Input: dimensioned drawing with shaded views. Units: mm. Origin: part minimum x, y, z. Coordinates: 2 decimals unless noted, no trailing zeros. Loops run counter-clockwise (first coordinate to the right, second up) from the corner with the lowest first, then second, coordinate; pieces in that order, holes last.
(1) Section A-A, the plane z = 21. Return loops of the section in (x, y) (1 decimal), then the cut area to 3 significant figures.
(2) Section C-C, the plane y = 2.65. Return loops of the section in (x, z) (1 decimal), then the cut area to 3 significant figures.
(3) Line query: L1, parallel to X at y = 2.6, z = 26; L2, parallel to X at y = 0.7, z = 24.5 (1 decimal); L3, parallel to Y at x = 32, z = 2. Output: solid intervals per line, ascending.
(4) Contact query for flat-ended pins moving along their axis: P1, Ø1.5, axis at y = 1.5, z = 5.5, coming from the +X side; P2, Ø1.1, axis at y = 2.5, z = 50, coming from the -X side. Output: stop coordinate, or through.
(5) Section B-B, the plane x = 47. Return loops of the section in (y, z) (1 decimal).
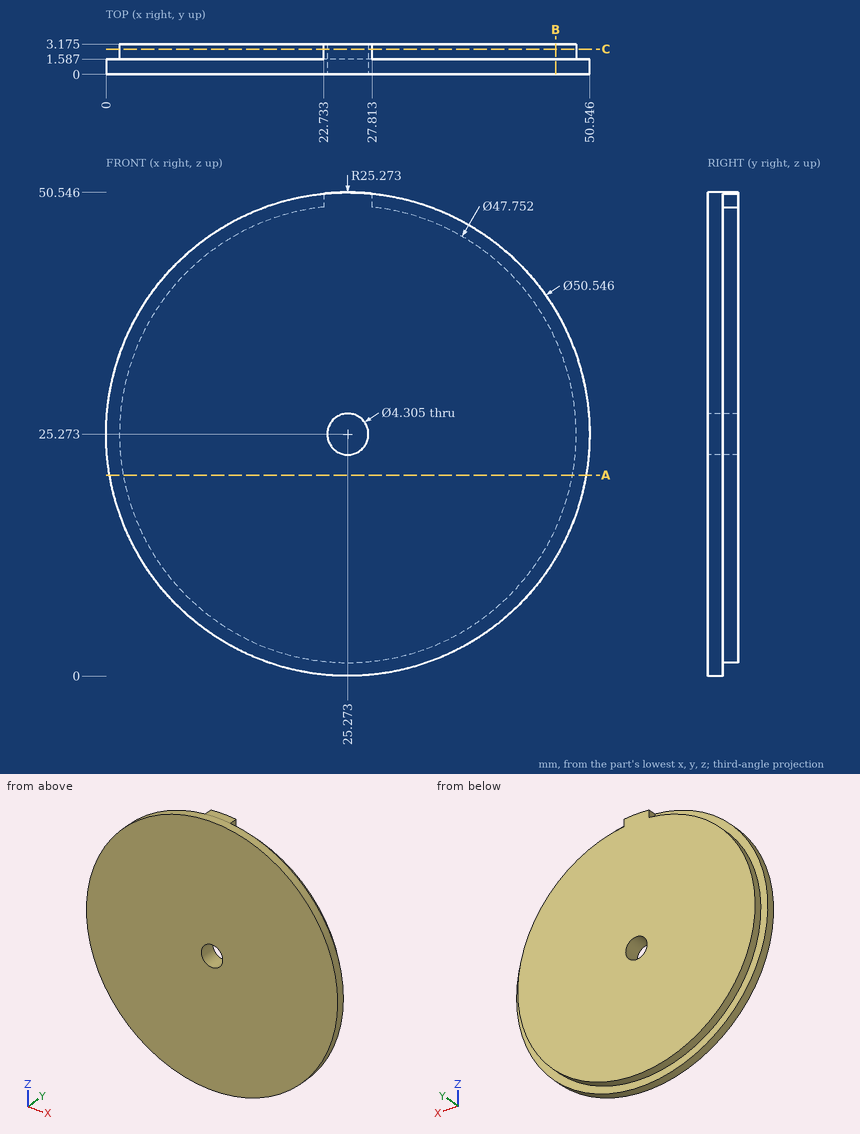
Report:
1. outline: (0.4, 0) - (50.2, 0) - (50.2, 1.6) - (48.8, 1.6) - (48.8, 3.2) - (1.8, 3.2) - (1.8, 1.6) - (0.4, 1.6) - close
1. area: 154 mm2
2. outline: (22.7, 49) arc R23.9 ccw (long way) to (27.8, 49) - (27.8, 50.4) arc R25.3 ccw to (22.7, 50.4) - close; hole circle Ø4.3 at (25.3, 25.3)
2. area: 1,780 mm2
3. L1: x = 1.41 to 23.25, 27.3 to 49.14
3. L2: x = 0 to 23.3, 27.3 to 50.5
3. L3: y = 0 to 1.59
4. P1: stops at x = 41.91
4. P2: stops at x = 22.73
5. outline: (0, 12.4) - (1.6, 12.4) - (1.6, 15.4) - (3.2, 15.4) - (3.2, 35.2) - (1.6, 35.2) - (1.6, 38.2) - (0, 38.2) - close
